```python
from build123d import *

# Parameters (mm, degrees)
SKETCH3_W           = 38.1
SKETCH3_H           = 38.1
SKETCH3_R           = 1.125
BOSS_EXTRUDE1_DEPTH = 2.5
BOSS_EXTRUDE2_START = 3
SKETCH2_R           = 1.125
BOSS_EXTRUDE2_DEPTH = 3
SKETCH4_W           = 8.75
SKETCH4_H           = 5.25
CUT_EXTRUDE1_DEPTH  = 10
SKETCH6_W           = 8.75
SKETCH6_H           = 2.75
CUT_EXTRUDE2_DEPTH  = 10
SKETCH7_R           = 0.9
BOSS_EXTRUDE3_DEPTH = 1.4


with BuildPart() as part:
    # Sketch3 → Boss-Extrude1 (new body)
    with BuildSketch(Plane.XY):
        with Locations((0.466348003, 11.564505911)):
            Rectangle(SKETCH3_W, SKETCH3_H)
        with Locations((-13.533651997, 25.564505911)):
            Circle(SKETCH3_R, mode=Mode.SUBTRACT)
        with Locations((14.466348003, 25.564505911)):
            Circle(SKETCH3_R, mode=Mode.SUBTRACT)
        with Locations((14.466348003, -2.435494089)):
            Circle(SKETCH3_R, mode=Mode.SUBTRACT)
        with Locations((-13.533651997, -2.435494089)):
            Circle(SKETCH3_R, mode=Mode.SUBTRACT)
    extrude(amount=-BOSS_EXTRUDE1_DEPTH)

    # Sketch2 → Boss-Extrude2 (add)
    # profile 1 of 4: a face of its own
    with BuildSketch(Plane.XY.offset(BOSS_EXTRUDE2_START)):
        with BuildLine():
            Line((-18.583651997, 30.614505911), (-10.333651997, 30.614505911))
            Line((-10.333651997, 30.614505911), (-10.333651997, 26.364505911))
            ThreePointArc((-10.333651997, 26.364505911), (-11.505224872, 23.536078787), (-14.333651997, 22.364505911))
            Line((-14.333651997, 22.364505911), (-18.583651997, 22.364505911))
            Line((-18.583651997, 22.364505911), (-18.583651997, 30.614505911))
        make_face()
        with Locations((-13.533651997, 25.564505911)):
            Circle(SKETCH2_R, mode=Mode.SUBTRACT)
    # profile 2 of 4: a face of its own
    with BuildSketch(Plane.XY.offset(BOSS_EXTRUDE2_START)):
        with BuildLine():
            Line((19.516348003, 30.614505911), (11.266348003, 30.614505911))
            Line((11.266348003, 30.614505911), (11.266348003, 26.364505911))
            ThreePointArc((11.266348003, 26.364505911), (12.437920878, 23.536078787), (15.266348003, 22.364505911))
            Line((15.266348003, 22.364505911), (19.516348003, 22.364505911))
            Line((19.516348003, 22.364505911), (19.516348003, 30.614505911))
        make_face()
        with Locations((14.466348003, 25.564505911)):
            Circle(SKETCH2_R, mode=Mode.SUBTRACT)
    # profile 3 of 4: a face of its own
    with BuildSketch(Plane.XY.offset(BOSS_EXTRUDE2_START)):
        with BuildLine():
            Line((19.516348003, -7.485494089), (11.266348003, -7.485494089))
            Line((11.266348003, -7.485494089), (11.266348003, -3.235494089))
            ThreePointArc((11.266348003, -3.235494089), (12.437920878, -0.407066964), (15.266348003, 0.764505911))
            Line((15.266348003, 0.764505911), (19.516348003, 0.764505911))
            Line((19.516348003, 0.764505911), (19.516348003, -7.485494089))
        make_face()
        with Locations((14.466348003, -2.435494089)):
            Circle(SKETCH2_R, mode=Mode.SUBTRACT)
    # profile 4 of 4: a face of its own
    with BuildSketch(Plane.XY.offset(BOSS_EXTRUDE2_START)):
        with BuildLine():
            Line((-18.583651997, -7.485494089), (-10.333651997, -7.485494089))
            Line((-10.333651997, -7.485494089), (-10.333651997, -3.235494089))
            ThreePointArc((-10.333651997, -3.235494089), (-11.505224872, -0.407066964), (-14.333651997, 0.764505911))
            Line((-14.333651997, 0.764505911), (-18.583651997, 0.764505911))
            Line((-18.583651997, 0.764505911), (-18.583651997, -7.485494089))
        make_face()
        with Locations((-13.533651997, -2.435494089)):
            Circle(SKETCH2_R, mode=Mode.SUBTRACT)
    extrude(amount=-BOSS_EXTRUDE2_DEPTH)

    # Sketch4 → Cut-Extrude1 (cut)
    with BuildSketch(Plane(origin=(0, 0, -2.5), x_dir=(-1, 0, 0), z_dir=(0, 0, -1))):
        with Locations((6.563651997, -2.110494089)):
            Rectangle(SKETCH4_W, SKETCH4_H)
    extrude(amount=-CUT_EXTRUDE1_DEPTH, mode=Mode.SUBTRACT)

    # Sketch6 → Cut-Extrude2 (cut)
    with BuildSketch(Plane(origin=(0, 0, -2.5), x_dir=(-1, 0, 0), z_dir=(0, 0, -1))):
        with Locations((6.563651997, -6.110494089)):
            Rectangle(SKETCH6_W, SKETCH6_H)
    extrude(amount=-CUT_EXTRUDE2_DEPTH, mode=Mode.SUBTRACT)

    # Sketch7 → Boss-Extrude3 (add)
    with BuildSketch(Plane.XY.offset(3)):
        with Locations((-16.533651997, 28.564505911)):
            Circle(SKETCH7_R)
        with Locations(Location((17.466348003, 28.564505911, 0), (0, 0, 180))):
            Circle(SKETCH7_R)
        with Locations((17.466348003, -5.435494089)):
            Circle(SKETCH7_R)
        with Locations(Location((-16.533651997, -5.435494089, 0), (0, 0, 180))):
            Circle(SKETCH7_R)
    extrude(amount=BOSS_EXTRUDE3_DEPTH)


solid = part.part
```
For this review, take the finished solid that the model builds, in its own axes (mm). A direction names the side the tool comes from. Coordinates: 2 decimals unless noted, no trailing zeros. Write each loop counter-clockwise with the first axis right and the second up, starting at its lowest first coordinate (ties: lowest second). Pieces come first, ordered by that corner, then holes.
(1) The part is to be moulded in two halves that separate along Y. For faces 1 (the face through (-12.37, 0.25, 1.52)), 2 (the face through (17, 29, 4.4)), 3 (the face through (-15, -7.485, 0)), say which applies: +Y half, -Y half, draft (parallel to the pull), parting line (faces both ways), or undercut.
(2) Tool access review of faces 4 (the face through (17, 0.765, 2)), 5 (the face through (-14.658, -2.386, 0.288)), 6 (the face through (-10.334, 29, 2)), 7 (the face through (-17.39, -5.71, 3.69)): name each direction out of +Z, -Z, +X, -X, +Y, -Y from which nothing blocks a thin tool from reaching the whole face with its end or side.
(3) For pin 1 Ø3.5 at (x, y) = (-13.53, 25.56) entering from +Z; pin 2 Ø4 at (x, z) = (-1.5, 3) entering from +Y; pin 3 Ø1.5 at (x, y) = (15, 18.5) entering from +Z, all flat-tipped, find the tip position at first contact; note any pin that passes through.
(4) Add section D-D on z = 3.75. Give the boundary of the cut face in (x, y).
(5) Add section C-C on y = 14.5. Give the boundary of the cut face in (x, z).
(6) Add section A-A on z = 1.75. Count the separate pieces of the cut face and the enclosed holes in it, then the cut area to 3 significant figures.
(7) Wall thickness on probe 1 along Y at (x, z) = (-13, 1); probe 2 along Z at (x, y) = (5.5, 22); probe 3 along Z at (x, y) = (13, 24.5): over which ranges is each line inside the solid? List them lowest first.
Answer sheet:
1. face 1: undercut
1. face 2: draft
1. face 3: -Y half
2. face 4: +Z, +X, -X
2. face 5: +Z, -Z
2. face 6: +Z, +Y, -Y
2. face 7: +Z
3. pin 1: stops at z = 3
3. pin 2: passes through
3. pin 3: stops at z = 0
4. outline: circle Ø1.8 at (-16.53, -5.44); circle Ø1.8 at (-16.53, 28.56); circle Ø1.8 at (17.47, -5.44); circle Ø1.8 at (17.47, 28.56)
5. outline: (-18.58, -2.5) - (19.52, -2.5) - (19.52, 0) - (-18.58, 0) - close
6. separate pieces: 4
6. enclosed holes: 4
6. area: 239 mm2
7. probe 1: y = -7.49 to -3.43, -1.45 to 0.54, 22.59 to 24.57, 26.55 to 30.61
7. probe 2: z = -2.5 to 0
7. probe 3: z = -2.5 to 3
